The listing builds one solid part. Answer for the finished solid, in the listing's coordinates (mm). A direction names the side the tool comes from. Round coordinates to 2 decimals unless told otherwise and drop trailing zeros. Loops run counter-clockwise (first coordinate to the right, second up) from the corner with the lowest first, then second, coordinate; pieces in that order, holes last. Notation, with made-up numbers: (52, 20) -> (100, 20) arc R13 ccw to (100, 37) -> close; hole circle Ø6 at (-27, 12.25). An arc over 180 degrees is marked (long way). Use a Markdown table: item, result. Add a question column.
Q1. Section C-C on z = 1.5 is taken. Give the vertices of the cut face in (x, y).
Q2. For a pull along Y with two mould halves and no side action, classify faces 1 (the flat face through (0, 36, 3)), 2 (the flat face through (54.108, -1, 3)), 3 (the flat face through (45, 47, 3)) as released by +Y, released by -Y, zero draft, split by the parting line, or undercut.
Q3. Given pin 1 Ø1.9 at (x, z) = (12, 4) entering from +Y; pin 2 Ø5 at (x, y) = (-39.5, 33.5) entering from -Z, each flat-ended and moving along its own axis, determine where each tip first touches the part or whether it passes through.
Q4. Which of the six approach directions +Z, -Z, +X, -X, +Y, -Y give full straight-line access (tool end or side, diameter ignored) to faces 4 (the cylindrical face through (-35.18, 35.25, 3.13)), 5 (the cylindrical face through (53.356, 46.287, 3.131)), 6 (the flat face through (-9, -42, 3)), 7 (the flat face through (-8, 42, 3))?
Q5. Section B-B on y = -30 is taken. Give the vertices of the cut face in (x, z), then the cut area to 3 significant figures.
Q6. Consider line 1 (Y direction, x = -29.5, z = 2.25); line 2 (X direction, y = 23.5, z = 5.5); line 3 (X direction, y = 41, z = 2.5). Determine where each line is inside the solid, lowest interval first.
Q7. Section D-D on y = -11 is taken. Give the vertices of the cut face in (x, z).
Q8. Section A-A on x = -15 is taken. Give the vertices of the cut face in (y, z), then the cut area to 3 significant figures.
from build123d import *

# Parameters (mm, degrees)
SKETCH1_R           = 2.25
SKETCH1_R_2         = 2
SKETCH1_W           = 72
SKETCH1_H           = 72
BOSS_EXTRUDE1_DEPTH = 6.35
FILLET1_START       = -1
FILLET1_DEPTH       = 8
FILLET1_2_DEPTH     = 6.35


with BuildPart() as part:
    # Sketch1 → Boss-Extrude1 (new body)
    with BuildSketch(Plane.XY):
        Polygon((54.107594743, 42), (54.107594743, 47), (36.107594743, 47), (36.107594743, 42), (-53.892405257, 42), (-53.892405257, -42), (36.107594743, -42), (36.107594743, -47), (54.107594743, -47), (54.107594743, -42), align=None)
        with Locations((-44.892405257, 30)):
            Circle(SKETCH1_R, mode=Mode.SUBTRACT)
        with Locations((45.107594743, 30)):
            Circle(SKETCH1_R, mode=Mode.SUBTRACT)
        with Locations((45.107594743, -30)):
            Circle(SKETCH1_R, mode=Mode.SUBTRACT)
        with Locations((-44.892405257, -30)):
            Circle(SKETCH1_R, mode=Mode.SUBTRACT)
        with Locations((45.107594743, -41)):
            Circle(SKETCH1_R_2, mode=Mode.SUBTRACT)
        with Locations(Location((45.107594743, 41, 0), (0, 0, 180))):
            Circle(SKETCH1_R_2, mode=Mode.SUBTRACT)
        with Locations((0.107594743, 0)):
            Rectangle(SKETCH1_W, SKETCH1_H, mode=Mode.SUBTRACT)
    extrude(amount=BOSS_EXTRUDE1_DEPTH)

    # Fillet1: read off the stored shape, not the designer's step
    # Fillet1 outline → Fillet1 (cut)
    with BuildSketch(Plane.XY.offset(FILLET1_START)):
        with BuildLine():
            Line((36.107594743, 47), (36.107594743, 44.5))
            ThreePointArc((36.107594743, 44.5), (36.83982779, 46.267766953), (38.607594743, 47))
            Line((38.607594743, 47), (36.107594743, 47))
        make_face()
        with BuildLine():
            Line((54.107594743, 47), (51.607594743, 47))
            ThreePointArc((51.607594743, 47), (53.375361696, 46.267766953), (54.107594743, 44.5))
            Line((54.107594743, 44.5), (54.107594743, 47))
        make_face()
        with BuildLine():
            ThreePointArc((-53.892405257, 39.5), (-53.16017221, 41.267766953), (-51.392405257, 42))
            Line((-51.392405257, 42), (-53.892405257, 42))
            Line((-53.892405257, 42), (-53.892405257, 39.5))
        make_face()
        with BuildLine():
            Line((54.107594743, -47), (54.107594743, -44.5))
            ThreePointArc((54.107594743, -44.5), (53.375361696, -46.267766953), (51.607594743, -47))
            Line((51.607594743, -47), (54.107594743, -47))
        make_face()
        with BuildLine():
            ThreePointArc((-51.392405257, -42), (-53.16017221, -41.267766953), (-53.892405257, -39.5))
            Line((-53.892405257, -39.5), (-53.892405257, -42))
            Line((-53.892405257, -42), (-51.392405257, -42))
        make_face()
        with BuildLine():
            Line((36.107594743, -47), (38.607594743, -47))
            ThreePointArc((38.607594743, -47), (36.83982779, -46.267766953), (36.107594743, -44.5))
            Line((36.107594743, -44.5), (36.107594743, -47))
        make_face()
    extrude(amount=FILLET1_DEPTH, mode=Mode.SUBTRACT)

    # Fillet1 2 outline → Fillet1 2 (add)
    with BuildSketch(Plane.XY):
        with BuildLine():
            ThreePointArc((36.107594743, -33.5), (35.375361696, -35.267766953), (33.607594743, -36))
            Line((33.607594743, -36), (36.107594743, -36))
            Line((36.107594743, -36), (36.107594743, -33.5))
        make_face()
        with BuildLine():
            Line((-35.892405257, -36), (-33.392405257, -36))
            ThreePointArc((-33.392405257, -36), (-35.16017221, -35.267766953), (-35.892405257, -33.5))
            Line((-35.892405257, -33.5), (-35.892405257, -36))
        make_face()
        with BuildLine():
            ThreePointArc((33.607594743, 36), (35.375361696, 35.267766953), (36.107594743, 33.5))
            Line((36.107594743, 33.5), (36.107594743, 36))
            Line((36.107594743, 36), (33.607594743, 36))
        make_face()
        with BuildLine():
            Line((-35.892405257, 36), (-35.892405257, 33.5))
            ThreePointArc((-35.892405257, 33.5), (-35.16017221, 35.267766953), (-33.392405257, 36))
            Line((-33.392405257, 36), (-35.892405257, 36))
        make_face()
        with BuildLine():
            Line((36.107594743, 42), (36.107594743, 44.5))
            ThreePointArc((36.107594743, 44.5), (35.375361696, 42.732233047), (33.607594743, 42))
            Line((33.607594743, 42), (36.107594743, 42))
        make_face()
        with BuildLine():
            Line((36.107594743, -42), (33.607594743, -42))
            ThreePointArc((33.607594743, -42), (35.375361696, -42.732233047), (36.107594743, -44.5))
            Line((36.107594743, -44.5), (36.107594743, -42))
        make_face()
    extrude(amount=FILLET1_2_DEPTH)


solid = part.part
Checked values:
| question | item | result |
|---|---|---|
| 1 | outline | (-53.89, -39.5) arc R2.5 ccw to (-51.39, -42) -> (33.61, -42) arc R2.5 cw to (36.11, -44.5) arc R2.5 ccw to (38.61, -47) -> (51.61, -47) arc R2.5 ccw to (54.11, -44.5) -> (54.11, 44.5) arc R2.5 ccw to (51.61, 47) -> (38.61, 47) arc R2.5 ccw to (36.11, 44.5) arc R2.5 cw to (33.61, 42) -> (-51.39, 42) arc R2.5 ccw to (-53.89, 39.5) -> close; hole circle Ø4.5 at (-44.89, -30); hole circle Ø4.5 at (-44.89, 30); hole (-35.89, -33.5) arc R2.5 ccw to (-33.39, -36) -> (33.61, -36) arc R2.5 ccw to (36.11, -33.5) -> (36.11, 33.5) arc R2.5 ccw to (33.61, 36) -> (-33.39, 36) arc R2.5 ccw to (-35.89, 33.5) -> close; hole circle Ø4.5 at (45.11, -30); hole circle Ø4.5 at (45.11, 30); hole circle Ø4 at (45.11, -41); hole circle Ø4 at (45.11, 41) |
| 2 | face 1 | undercut |
| 2 | face 2 | zero draft |
| 2 | face 3 | released by +Y |
| 3 | pin 1 | stops at y = 42 |
| 3 | pin 2 | stops at z = 0 |
| 4 | face 4 | +Z, -Z |
| 4 | face 5 | +Z, -Z, +X, +Y |
| 4 | face 6 | +Z, -Z, -X, -Y |
| 4 | face 7 | +Z, -Z, -X, +Y |
| 5 | outline | (-53.89, 0) -> (-47.14, 0) -> (-47.14, 6.35) -> (-53.89, 6.35) -> close; (-42.64, 0) -> (-35.89, 0) -> (-35.89, 6.35) -> (-42.64, 6.35) -> close; (36.11, 0) -> (42.86, 0) -> (42.86, 6.35) -> (36.11, 6.35) -> close; (47.36, 0) -> (54.11, 0) -> (54.11, 6.35) -> (47.36, 6.35) -> close |
| 5 | area | 171 mm2 |
| 6 | line 1 | y = -42 to -36, 36 to 42 |
| 6 | line 2 | x = -53.89 to -35.89, 36.11 to 54.11 |
| 6 | line 3 | x = -53.39 to 43.11, 47.11 to 54.11 |
| 7 | outline | (-53.89, 0) -> (-35.89, 0) -> (-35.89, 6.35) -> (-53.89, 6.35) -> close; (36.11, 0) -> (54.11, 0) -> (54.11, 6.35) -> (36.11, 6.35) -> close |
| 8 | outline | (-42, 0) -> (-36, 0) -> (-36, 6.35) -> (-42, 6.35) -> close; (36, 0) -> (42, 0) -> (42, 6.35) -> (36, 6.35) -> close |
| 8 | area | 76.2 mm2 |
